Geometry: final body of the model. Coordinates: model frame, mm. A direction names the side the tool comes from. Round coordinates to 2 decimals unless told otherwise and drop trailing zeros. Loops run counter-clockwise (first coordinate to the right, second up) from the corner with the lowest first, then second, coordinate; pieces in that order, holes last. Notation, with made-up numbers: (-1, 55) - (37, 55) arc R14 cw to (37, 74) - close; hole circle Ø3 at (18.25, 39). An arc over 180 degrees is marked (long way). Use CSV: the item, a comma, the result in double quotes.
from build123d import *

# Parameters (mm, degrees)
SKETCH036_W  = 19.99996
SKETCH036_H  = 23.09876
SKETCH036_R  = 1.7
PAD003_DEPTH = 2.54
SKETCH051_W  = 19.99996
SKETCH051_H  = 8.89
SKETCH051_R  = 1.7
PAD_DEPTH    = 12.7
SKETCH050_R  = 0.9
PAD011_DEPTH = 2.975
SKETCH_R     = 1.5875
POCKET_DEPTH = 8.89
FILLET_R     = 1.00076


with BuildPart() as part:
    # Sketch036 → Pad003 (new body)
    with BuildSketch(Plane(origin=(0, 10, -45.999574), x_dir=(-1, 0, 0), z_dir=(0, 1, 0))):
        with Locations((0, 1.15062)):
            Rectangle(SKETCH036_W, SKETCH036_H)
        with Locations((-7.5, 5.00124)):
            Circle(SKETCH036_R, mode=Mode.SUBTRACT)
        with Locations((-7.5, -4.99876)):
            Circle(SKETCH036_R, mode=Mode.SUBTRACT)
        with Locations((7.5, -4.99876)):
            Circle(SKETCH036_R, mode=Mode.SUBTRACT)
        with Locations((7.5, 5.00124)):
            Circle(SKETCH036_R, mode=Mode.SUBTRACT)
    extrude(amount=PAD003_DEPTH)

    # Sketch051 (on Face10 of Pad003) → Pad (join)
    with BuildSketch(Plane(origin=(0, 12.54, -45.999574), x_dir=(-1, 0, 0), z_dir=(0, 1, 0))):
        with Locations((0, 5.00124)):
            Rectangle(SKETCH051_W, SKETCH051_H)
        with Locations((-7.5, 5.00124)):
            Circle(SKETCH051_R, mode=Mode.SUBTRACT)
        with Locations((7.5, 5.00124)):
            Circle(SKETCH051_R, mode=Mode.SUBTRACT)
    extrude(amount=PAD_DEPTH)

    # Sketch050 → Pad011 (join)
    with BuildSketch(Plane(origin=(0, 10, -56.398334), x_dir=(-1, 0, 0), z_dir=(0, 0, -1))):
        with BuildLine():
            Line((-3.175, 2.54), (-3.175, 0))
            Line((-3.175, 0), (3.175, 0))
            Line((3.175, 0), (3.175, 2.54))
            Line((3.175, 2.54), (1.90374, 6.488023))
            ThreePointArc((1.90374, 6.488023), (0, 7.87502), (-1.90374, 6.488023))
            Line((-1.90374, 6.488023), (-3.175, 2.54))
        make_face()
        with Locations((0, 5.87502)):
            Circle(SKETCH050_R, mode=Mode.SUBTRACT)
    extrude(amount=-PAD011_DEPTH)

    # Sketch (on Face16 of Pad011) → Pocket (cut)
    with BuildSketch(Plane(origin=(0, 10, -36.553334), x_dir=(1, 0, 0), z_dir=(0, 0, 1))):
        with Locations((0, 5.87502)):
            Circle(SKETCH_R)
    extrude(amount=-POCKET_DEPTH, mode=Mode.SUBTRACT)

    # Fillet
    fillet_edges = [part.edges().sort_by_distance(p)[0] for p in [
        (-1.5875, 15.87502, -36.553334),
        (-1.5875, 15.87502, -45.443334),
        (9.99998, 11.27, -33.299574),
        (-9.99998, 11.27, -33.299574),
        (9.99998, 11.27, -56.398334),
        (-9.99998, 11.27, -56.398334),
    ]]
    fillet(fillet_edges, radius=FILLET_R)


solid = part.part
Item 1: Mould query, pull axis Z, two halves, no side actions, for faces 5 (the flat face through (-2.548, 14.486, -54.932)), 6 (the cylindrical face through (9.715, 11.288, -33.601)), 7 (the flat face through (0, 14.7, -53.423)). Classes: released by +Z, released by -Z, zero draft, split by the parting line, or undercut.
Final values:
face 5,"zero draft"
face 6,"released by +Z"
face 7,"undercut"
Item 2: Material intervals for line 1 (Z direction, x = -7.5, y = 11.7); line 2 (Z direction, x = 7.5, y = 21.25); line 3 (Y direction, x = 0, z = -54.5), sorted ascending.
Final values:
line 1,"z = -56.4 to -52.7, -49.3 to -42.7, -39.3 to -33.3"
line 2,"z = -45.44 to -42.7, -39.3 to -36.55"
line 3,"y = 10 to 14.98, 16.78 to 17.88"
Item 3: Section C-C on x = 0. Return the cut outline in (y, z).
Final values:
outline,"(10, -56.4) - (14.98, -56.4) - (14.98, -53.42) - (12.54, -53.42) - (12.54, -45.44) - (13.29, -45.44) arc R1 ccw to (14.29, -44.44) - (14.29, -37.55) arc R1 ccw to (13.29, -36.55) - (12.54, -36.55) - (12.54, -33.3) - (10, -33.3) - close; (16.78, -56.4) - (17.88, -56.4) - (17.88, -53.42) - (16.78, -53.42) - close; (17.46, -44.44) arc R1 ccw to (18.46, -45.44) - (25.24, -45.44) - (25.24, -36.55) - (18.46, -36.55) arc R1 ccw to (17.46, -37.55) - close"
Item 4: Reachability of faces 1 (the flat face through (0, 12.54, -35)), 2 (the cylindrical face through (-0.035, 17.875, -54.932)), 3 (the flat face through (2.53, 14.54, -54.93)), 4 (the cylindrical face through (-9.699, 11.288, -33.585)) from +Z, -Z, +X, -X, +Y, -Y: full face, straight path, thin tool, end or side. Return the list, or none.
Final values:
face 1,"+Z, +X, -X, +Y"
face 2,"-Z, +Y"
face 3,"-Z, +X, +Y"
face 4,"+Z, -X, +Y, -Y"
Item 5: Section B-B on x = -5. Return the cut outline in (y, z).
Final values:
outline,"(10, -56.4) - (12.54, -56.4) - (12.54, -45.44) - (25.24, -45.44) - (25.24, -36.55) - (12.54, -36.55) - (12.54, -33.3) - (10, -33.3) - close"
Item 6: Section D-D on y = 21.75. Return the cut outline in (x, z), plus the area to 3 significant figures.
Final values:
outline,"(-10, -45.44) - (10, -45.44) - (10, -36.55) - (-10, -36.55) - close; hole circle Ø3.4 at (-7.5, -41); hole circle Ø3.4 at (7.5, -41)"
area,"160 mm²"
Item 7: Pin query (flat end, axial travel): P1, Ø2.5, axis at x = -7.5, z = -51, coming from the +Y side; P2, Ø4.5, axis at x = -7.5, z = -41, coming from the -Y side; P3, Ø1.5, axis at x = -6.5, y = 23.5, coming from the +Z side; P4, Ø3, axis at x = -3.5, z = -51.5, coming from the +Y side. Return the tip coordinate at first contact, or that it passes through.
Final values:
P1,"passes through"
P2,"stops at y = 10"
P3,"stops at z = -36.55"
P4,"stops at y = 12.54"
Item 8: Section A-A on x = 7.5. Return the cut outline in (y, z).
Final values:
outline,"(10, -56.4) - (12.54, -56.4) - (12.54, -52.7) - (10, -52.7) - close; (10, -49.3) - (12.54, -49.3) - (12.54, -45.44) - (25.24, -45.44) - (25.24, -42.7) - (10, -42.7) - close; (10, -39.3) - (25.24, -39.3) - (25.24, -36.55) - (12.54, -36.55) - (12.54, -33.3) - (10, -33.3) - close"
